```python
from build123d import *

# Parameters (mm, degrees)
SKETCH3_W           = 35
SKETCH3_H           = 27
SKETCH3_R           = 1.65
BOSS_EXTRUDE2_DEPTH = 4
SKETCH5_W           = 35
SKETCH5_H           = 2
BOSS_EXTRUDE3_DEPTH = 6
SKETCH7_R           = 1.65
CUT_EXTRUDE2_DEPTH  = 4
CUT_EXTRUDE3_DEPTH  = 2.6
SKETCH9_R           = 2.7
CUT_EXTRUDE4_DEPTH  = 3
SKETCH10_W          = 1.2
SKETCH10_H          = 2.8
CUT_EXTRUDE5_DEPTH  = 4
SKETCH11_W          = 6
SKETCH11_H          = 2.8
CUT_EXTRUDE6_DEPTH  = 1


with BuildPart() as part:
    # Sketch3 → Boss-Extrude2 (new body)
    with BuildSketch(Plane(origin=(0, 0, 0), x_dir=(1, 0, 0), z_dir=(0, 1, 0))):
        Rectangle(SKETCH3_W, SKETCH3_H)
        with Locations(Location((10, -1.2, 0), (0, 0, 270))):
            Circle(SKETCH3_R, mode=Mode.SUBTRACT)
        with Locations(Location((-10, -1.2, 0), (0, 0, 90))):
            Circle(SKETCH3_R, mode=Mode.SUBTRACT)
    extrude(amount=BOSS_EXTRUDE2_DEPTH)

    # Sketch5 → Boss-Extrude3 (add)
    with BuildSketch(Plane(origin=(0, 4, 0), x_dir=(1, 0, 0), z_dir=(0, 1, 0))):
        with Locations((0, -12.5)):
            Rectangle(SKETCH5_W, SKETCH5_H)
    extrude(amount=BOSS_EXTRUDE3_DEPTH)

    # Sketch7 → Cut-Extrude2 (cut)
    with BuildSketch(Plane.XZ):
        with Locations(Location((-13.25, -9.25, 0), (0, 0, 270))):
            Circle(SKETCH7_R)
        with Locations(Location((-13.25, 6.75, 0), (0, 0, 270))):
            Circle(SKETCH7_R)
    extrude(amount=-CUT_EXTRUDE2_DEPTH, mode=Mode.SUBTRACT)

    # Sketch8 → Cut-Extrude3 (cut)
    with BuildSketch(Plane(origin=(0, 4, 0), x_dir=(1, 0, 0), z_dir=(0, 1, 0))):
        Polygon((-10.45, 7.633419246), (-10.45, 10.866580754), (-13.25, 12.483161507), (-16.05, 10.866580754), (-16.05, 7.633419246), (-13.25, 6.016838493), align=None)
        Polygon((-10.45, -5.133419246), (-13.25, -3.516838493), (-16.05, -5.133419246), (-16.05, -8.366580754), (-13.25, -9.983161507), (-10.45, -8.366580754), align=None)
    extrude(amount=-CUT_EXTRUDE3_DEPTH, mode=Mode.SUBTRACT)

    # Sketch9 → Cut-Extrude4 (cut)
    with BuildSketch(Plane.XZ):
        with Locations(Location((-10, 1.2, 0), (0, 0, 270))):
            Circle(SKETCH9_R)
        with Locations(Location((10, 1.2, 0), (0, 0, 270))):
            Circle(SKETCH9_R)
    extrude(amount=-CUT_EXTRUDE4_DEPTH, mode=Mode.SUBTRACT)

    # Sketch10 → Cut-Extrude5 (cut)
    with BuildSketch(Plane.XZ):
        with Locations((6.4, 8.219052272)):
            Rectangle(SKETCH10_W, SKETCH10_H)
        with Locations((13.6, 8.219052272)):
            Rectangle(SKETCH10_W, SKETCH10_H)
    extrude(amount=-CUT_EXTRUDE5_DEPTH, mode=Mode.SUBTRACT)

    # Sketch11 → Cut-Extrude6 (cut)
    with BuildSketch(Plane(origin=(0, 4, 0), x_dir=(1, 0, 0), z_dir=(0, 1, 0))):
        with Locations((10, -8.219052272)):
            Rectangle(SKETCH11_W, SKETCH11_H)
    extrude(amount=-CUT_EXTRUDE6_DEPTH, mode=Mode.SUBTRACT)


solid = part.part
```
Geometry check sheet. Reference: the model listing, model coordinates, mm. A direction names the side the tool comes from. Round coordinates to 2 decimals unless told otherwise and drop trailing zeros. Loops run counter-clockwise (first coordinate to the right, second up) from the corner with the lowest first, then second, coordinate; pieces in that order, holes last. Notation, with made-up numbers: (-28, 74.5) - (-13, 74.5) arc R22 ccw to (-13, 93.5) - close; hole circle Ø3 at (-4.75, -1.75). An arc over 180 degrees is marked (long way). Use a Markdown table: item, result.
Q1. Draft check along Z on faces 1 (the flat face through (0, 2, -13.5)), 2 (the flat face through (9.9, 3.3, 6.819)), 3 (the flat face through (0, 4, -1)). Enter one of: released by +Z, released by -Z, zero draft, split by the parting line, or undercut.
Solutions:
| item | result |
|---|---|
| face 1 | released by -Z |
| face 2 | undercut |
| face 3 | zero draft |
Q2. Cross-section at D-D on x = 4.5. Record the cut outline in (y, z).
Solutions:
| item | result |
|---|---|
| outline | (0, -13.5) - (4, -13.5) - (4, 11.5) - (10, 11.5) - (10, 13.5) - (0, 13.5) - close |
Q3. Cross-section at C-C on x = -10. Record the cut outline in (y, z).
Solutions:
| item | result |
|---|---|
| outline | (0, -13.5) - (4, -13.5) - (4, -0.45) - (3, -0.45) - (3, -1.5) - (0, -1.5) - close; (0, 3.9) - (3, 3.9) - (3, 2.85) - (4, 2.85) - (4, 11.5) - (10, 11.5) - (10, 13.5) - (0, 13.5) - close |
Q4. Cross-section at B-B on y = 2. Record the cut outline in (x, z).
Solutions:
| item | result |
|---|---|
| outline | (-17.5, -13.5) - (17.5, -13.5) - (17.5, 13.5) - (-17.5, 13.5) - close; hole (-16.05, -10.87) - (-13.25, -12.48) - (-10.45, -10.87) - (-10.45, -7.63) - (-13.25, -6.02) - (-16.05, -7.63) - close; hole (-16.05, 5.13) - (-13.25, 3.52) - (-10.45, 5.13) - (-10.45, 8.37) - (-13.25, 9.98) - (-16.05, 8.37) - close; hole circle Ø5.4 at (-10, 1.2); hole (5.8, 6.82) - (7, 6.82) - (7, 9.62) - (5.8, 9.62) - close; hole circle Ø5.4 at (10, 1.2); hole (13, 6.82) - (14.2, 6.82) - (14.2, 9.62) - (13, 9.62) - close |
Q5. Material ranges on line 1 (X direction, y = 0.85, z = 1.2); line 2 (Z direction, x = 10, y = 3.6); line 3 (Z direction, x = -13.5, y = 0.5), recorded low to high.
Solutions:
| item | result |
|---|---|
| line 1 | x = -17.5 to -12.7, -7.3 to 7.3, 12.7 to 17.5 |
| line 2 | z = -13.5 to -0.45, 2.85 to 6.82, 9.62 to 13.5 |
| line 3 | z = -13.5 to -10.88, -7.62 to 5.12, 8.38 to 13.5 |
Q6. Go/stop test with flat-tipped pins: P1, Ø4, axis at y = 4.5, z = 8.5, coming from the +X side; P2, Ø4, axis at x = -13.25, z = 6.75, coming from the +Y side; P3, Ø0.8, axis at x = 9.5, z = 9, coming from the +Y side; P4, Ø1.6, axis at x = 11, z = 0, coming from the -Y side. Record where each tip stops, or that it passes through.
Solutions:
| item | result |
|---|---|
| P1 | stops at x = 17.5 |
| P2 | stops at y = 1.4 |
| P3 | stops at y = 3 |
| P4 | stops at y = 3 |
Q7. Access from +Z, -Z, +X, -X, +Y, -Y to the whole of each face (thin tool, end or side, straight path). Record for faces 4 (the flat face through (14.2, 2, 8)), 5 (the flat face through (-17.5, 3, 0)), 6 (the flat face through (-11.83, 2.718, 4.336)).
Solutions:
| item | result |
|---|---|
| face 4 | +Y, -Y |
| face 5 | +Z, -Z, -X, +Y, -Y |
| face 6 | +Y |
Q8. Cross-section at A-A on z = -9.25. Record the cut outline in (x, y).
Solutions:
| item | result |
|---|---|
| outline | (-17.5, 0) - (-14.9, 0) - (-14.9, 1.4) - (-16.05, 1.4) - (-16.05, 4) - (-17.5, 4) - close; (-11.6, 0) - (17.5, 0) - (17.5, 4) - (-10.45, 4) - (-10.45, 1.4) - (-11.6, 1.4) - close |
